Geometry check sheet. Reference: the model listing, model coordinates, mm. Give positions to 0.01 mm unless a question says otherwise; leave off trailing zeros. Order: outer loops, then holes, each group sorted by start corner. A loop starts at its lowest first (then second) coordinate and runs counter-clockwise, first axis right, second up.
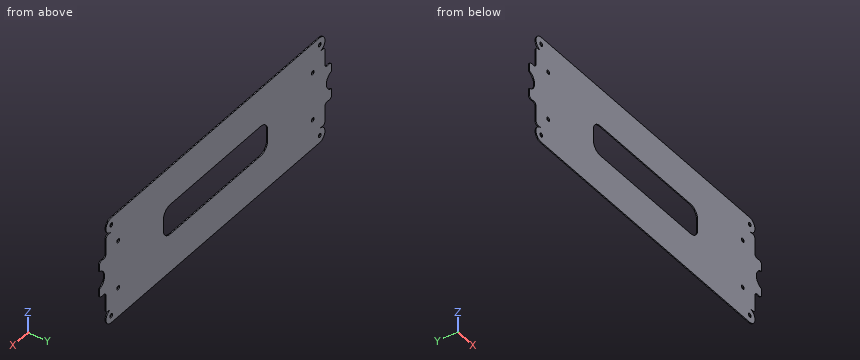
from build123d import *

# Parameters (mm, degrees)
SKETCH1_R           = 2
SKETCH1_W           = 150
SKETCH1_H           = 31.5
BOSS_EXTRUDE1_DEPTH = 1
FILLET1_R           = 10
FILLET2_R           = 3


with BuildPart() as part:
    # Sketch1 → Boss-Extrude1 (new body)
    with BuildSketch(Plane(origin=(0, 0, 0), x_dir=(1, 0, 0), z_dir=(0, 1, 0))):
        with BuildLine():
            Line((150, 55.75), (-150, 55.75))
            ThreePointArc((-150, 55.75), (-157.5, 48.25), (-150, 40.75))
            Line((-150, 40.75), (-154.5, 40.75))
            ThreePointArc((-154.5, 40.75), (-156.621320344, 39.871320344), (-157.5, 37.75))
            Line((-157.5, 37.75), (-157.5, 19))
            Line((-157.5, 19), (-167.025, 19))
            Line((-167.025, 19), (-167.025, 9.312659395))
            ThreePointArc((-167.025, 9.312659395), (-159.5, 0), (-167.025, -9.312659395))
            Line((-167.025, -9.312659395), (-167.025, -19))
            Line((-167.025, -19), (-157.5, -19))
            Line((-157.5, -19), (-157.5, -37.75))
            ThreePointArc((-157.5, -37.75), (-156.621320344, -39.871320344), (-154.5, -40.75))
            Line((-154.5, -40.75), (-150, -40.75))
            ThreePointArc((-150, -40.75), (-157.5, -48.25), (-150, -55.75))
            Line((-150, -55.75), (150, -55.75))
            ThreePointArc((150, -55.75), (157.5, -48.25), (150, -40.75))
            Line((150, -40.75), (154.5, -40.75))
            ThreePointArc((154.5, -40.75), (156.621320344, -39.871320344), (157.5, -37.75))
            Line((157.5, -37.75), (157.5, -19))
            Line((157.5, -19), (167.025, -19))
            Line((167.025, -19), (167.025, -9.312659395))
            ThreePointArc((167.025, -9.312659395), (159.5, 0), (167.025, 9.312659395))
            Line((167.025, 9.312659395), (167.025, 19))
            Line((167.025, 19), (157.5, 19))
            Line((157.5, 19), (157.5, 37.75))
            ThreePointArc((157.5, 37.75), (156.621320344, 39.871320344), (154.5, 40.75))
            Line((154.5, 40.75), (150, 40.75))
            ThreePointArc((150, 40.75), (157.5, 48.25), (150, 55.75))
        make_face()
        with Locations(Location((-150, 48.25, 0), (0, 0, 270))):
            Circle(SKETCH1_R, mode=Mode.SUBTRACT)
        with Locations(Location((150, 48.25, 0), (0, 0, 270))):
            Circle(SKETCH1_R, mode=Mode.SUBTRACT)
        with Locations(Location((150, -48.25, 0), (0, 0, 270))):
            Circle(SKETCH1_R, mode=Mode.SUBTRACT)
        with Locations(Location((-150, -48.25, 0), (0, 0, 270))):
            Circle(SKETCH1_R, mode=Mode.SUBTRACT)
        with Locations(Location((-140, 25, 0), (0, 0, 270))):
            Circle(SKETCH1_R, mode=Mode.SUBTRACT)
        with Locations(Location((-140, -25, 0), (0, 0, 270))):
            Circle(SKETCH1_R, mode=Mode.SUBTRACT)
        with Locations(Location((140, -25, 0), (0, 0, 270))):
            Circle(SKETCH1_R, mode=Mode.SUBTRACT)
        with Locations(Location((140, 25, 0), (0, 0, 270))):
            Circle(SKETCH1_R, mode=Mode.SUBTRACT)
        Rectangle(SKETCH1_W, SKETCH1_H, mode=Mode.SUBTRACT)
    extrude(amount=BOSS_EXTRUDE1_DEPTH)

    # Fillet1
    fillet1_edges = [part.edges().sort_by_distance(p)[0] for p in [
        (-75, 0.5, -15.75),
        (-75, 0.5, 15.75),
        (75, 0.5, 15.75),
        (75, 0.5, -15.75),
    ]]
    fillet(fillet1_edges, radius=FILLET1_R)

    # Fillet2
    fillet2_edges = [part.edges().sort_by_distance(p)[0] for p in [
        (-157.5, 0.5, 19),
        (-167.025, 0.5, 19),
        (-167.025, 0.5, -19),
        (-157.5, 0.5, -19),
        (157.5, 0.5, -19),
        (167.025, 0.5, -19),
        (167.025, 0.5, 19),
        (157.5, 0.5, 19),
    ]]
    fillet(fillet2_edges, radius=FILLET2_R)


solid = part.part
Item 1: Sectioned sample at C-C (y = 0.15). Give the number of separate pieces and of enclosed holes in the cut face, and give its area (3 significant figures).
Reported:
separate pieces: 1
enclosed holes: 9
area: 30,800 mm2
Item 2: Scan lines: L1, parallel to Z at x = -140, y = 0.4; L2, parallel to X at y = 0.4, z = 25; L3, parallel to Z at x = 31, y = 0.1. Record each from-to range of solid material in increasing order.
Reported:
L1: z = -55.75 to -27, -23 to 23, 27 to 55.75
L2: x = -157.5 to -142, -138 to 138, 142 to 157.5
L3: z = -55.75 to -15.75, 15.75 to 55.75
Item 3: Gauge pin test, flat ends, axial feed: pin 1 (0.5 mm diameter, centred on x = -163, y = 0.5, fed in from -Z); pin 2 (0.5 mm diameter, centred on y = 0.5, z = -30.5, fed in from -X). Record the tip position at first contact, or that the pin passes through.
Reported:
pin 1: stops at z = -19
pin 2: stops at x = -157.5
Item 4: Sectioned sample at A-A (x = 50). Enter the section's corners in (y, z), and give its area (3 significant figures).
Reported:
outline: (0, -55.75) - (1, -55.75) - (1, -15.75) - (0, -15.75) - close; (0, 15.75) - (1, 15.75) - (1, 55.75) - (0, 55.75) - close
area: 80.0 mm2
Item 5: Sectioned sample at B-B (z = -1). Enter the section's corners in (x, y).
Reported:
outline: (-159.55, 0) - (-75, 0) - (-75, 1) - (-159.55, 1) - close; (75, 0) - (159.55, 0) - (159.55, 1) - (75, 1) - close
